```python
from build123d import *

# Parameters (mm, degrees)
F0_W     = 87.1728
F0_H     = 50.038
F1_DEPTH = 7.366
F3_DEPTH = 2.54
F4_W     = 70.104
F4_H     = 10.922
F5_DEPTH = 5.08
F6_R     = 1.778
F7_DEPTH = 7.367


with BuildPart() as f1:
    # F0 (on Top) → F1 (new body)
    with BuildSketch(Plane.XY):
        with Locations((43.5864, 25.019)):
            Rectangle(F0_W, F0_H)
    extrude(amount=F1_DEPTH)

    # F2 (on face) → F3 (join)
    with BuildSketch(Plane.XY.offset(7.366)):
        Polygon((0, 37.106431), (0, 13.208), (87.1728, 13.208), (87.1728, 37.106431), (74.241231, 50.038), (12.931569, 50.038), align=None)
    extrude(amount=F3_DEPTH)

    # F4 (on face) → F5 (join)
    with BuildSketch(Plane.XY.offset(7.366)):
        with Locations((43.5864, 7.747)):
            Rectangle(F4_W, F4_H)
    extrude(amount=F5_DEPTH)

    # F6 (on face) → F7 (cut, through all)
    with BuildSketch(Plane.XY.offset(7.366)):
        with Locations((4.2926, 45.7454)):
            Circle(F6_R)
        with Locations((4.2926, 4.2926)):
            Circle(F6_R)
        with Locations((82.8802, 4.2926)):
            Circle(F6_R)
        with Locations((82.8802, 45.7454)):
            Circle(F6_R)
    extrude(amount=-F7_DEPTH, mode=Mode.SUBTRACT)


solid = f1.part
```
Model file for the job. Use its own axes, mm. A direction names the side the tool comes from. Coordinates: 2 decimals unless noted, no trailing zeros. Order: outer loops, then holes, each group sorted by start corner. A loop starts at its lowest first (then second) coordinate and runs counter-clockwise, first axis right, second up. Notation, with made-up numbers: (-14.75, -32.75) -> (19.25, -32.75) arc R18 ccw to (19.25, -2.75) -> close; hole circle Ø6 at (29, 19). An arc over 180 degrees is marked (long way). Answer as a JSON object with one key per item and string values. Group by question number.
1) Drill centre lines: L1, parallel to Z at x = 39.5, y = 45; L2, parallel to Y at x = 38, z = 9; L3, parallel to Z at x = 8, y = 46. Where is each one in solid material? Low to high.
2) Cut at A-A, the plane x = 26. Write the cut outline in (y, z).
3) Cut at B-B, the plane z = 8.75. Write the cut outline in (x, y), then the cut area to 3 significant figures.
4) Cut at D-D, the plane y = 30.5. Write the cut outline in (x, z), then the cut area to 3 significant figures.
5) Pull direction X, two halves, no side cores. Call faces 4 (the face through (4, 13.208, 9)), 5 (the face through (8.534, 8, 10)), 6 (the face through (84.576, 4.827, 3.735)), 7 (the face through (5.935, 3.612, 3.735)): +X half, -X half, draft (parallel to the pull), parting line (faces both ways), or undercut.
6) Flat gauge pins, fed straight in: pin 1 (2 mm diameter, centred on x = 60, z = 11.5, fed in from +Y); pin 2 (5.5 mm diameter, centred on y = 10, z = 10.5, fed in from +X); pin 3 (6.5 mm diameter, centred on x = 5.5, y = 44, fed in from +Z). Where does each tip first touch, or does it go through?
7) Which spindle directions (+Z, -Z, +X, -X, +Y, -Y) get a long thin tool onto all of the face, cutting with end or side? Do faces 1 (the face through (43, 32, 9.906)), 2 (the face through (85, 47, 7.366)), 3 (the face through (43, 2.286, 10)). Say none if no direction does.
8) Cut at C-C, the plane y = 38.5. Write the cut outline in (x, z).
Check values:
{
 "1": {"L1": "z = 0 to 9.91", "L2": "y = 2.29 to 50.04", "L3": "z = 0 to 7.37"},
 "2": {"outline": "(0, 0) -> (50.04, 0) -> (50.04, 9.91) -> (13.21, 9.91) -> (13.21, 12.45) -> (2.29, 12.45) -> (2.29, 7.37) -> (0, 7.37) -> close"},
 "3": {"outline": "(0, 13.21) -> (8.53, 13.21) -> (8.53, 2.29) -> (78.64, 2.29) -> (78.64, 13.21) -> (87.17, 13.21) -> (87.17, 37.11) -> (74.24, 50.04) -> (12.93, 50.04) -> (0, 37.11) -> close", "area": "3,810 mm²"},
 "4": {"outline": "(0, 0) -> (87.17, 0) -> (87.17, 9.91) -> (0, 9.91) -> close", "area": "864 mm²"},
 "5": {"face 4": "draft", "face 5": "-X half", "face 6": "undercut", "face 7": "undercut"},
 "6": {"pin 1": "stops at y = 13.21", "pin 2": "stops at x = 78.64", "pin 3": "stops at z = 9.91"},
 "7": {"face 1": "+Z, +X, -X, +Y", "face 2": "+Z, +X, +Y", "face 3": "+Z, +X, -X, -Y"},
 "8": {"outline": "(0, 0) -> (87.17, 0) -> (87.17, 7.37) -> (85.78, 7.37) -> (85.78, 9.91) -> (1.39, 9.91) -> (1.39, 7.37) -> (0, 7.37) -> close"}
}
